Design review of the part shown in the three views and the two pictorial views. Dimensions are in mm from the part's minimum x, y and z. A direction names the side the tool comes from. Give positions to 0.01 mm unless a question says otherwise; leave off trailing zeros. Order: outer loops, then holes, each group sorted by start corner. A loop starts at its lowest first (then second) coordinate and runs counter-clockwise, first axis right, second up. Notation, with made-up numbers: (-24.75, -12.75) - (-9.75, -12.75) arc R7 ccw to (-9.75, -6.75) - close; hole circle Ø5 at (80.25, 79.5). An arc over 180 degrees is marked (long way). Put each result on its own line as item: value.
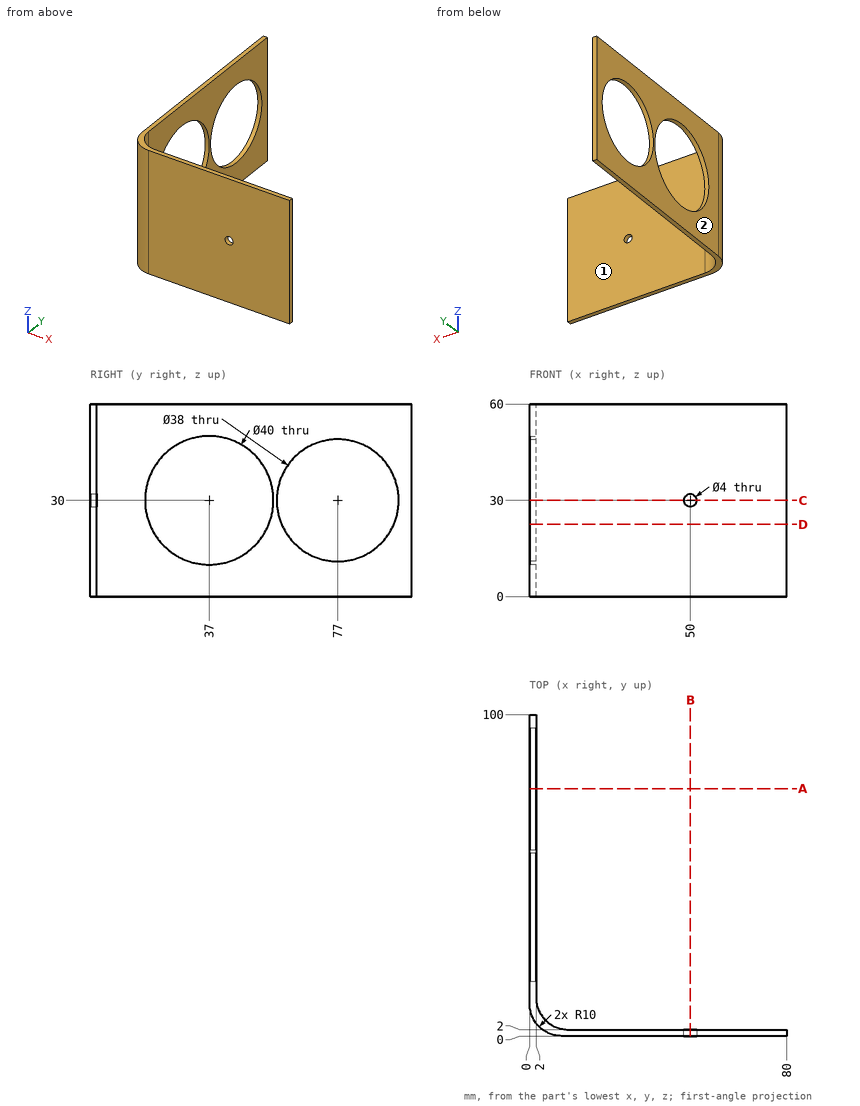
(1) Clearance check with flat-ended pins moving along their axes: pin 1 Ø1.5 at (x, z) = (29, 23) entering from -Y; pin 2 Ø18 at (y, z) = (49.5, 29.5) entering from +X; pin 3 Ø2 at (x, z) = (33, 8.5) entering from +Y. State where each tip first meets the part, or that it passes through.
The answers:
pin 1: y = 0
pin 2: x = 2
pin 3: y = 2
(2) Wall thickness on L1, parallel to Y at x = 1, z = 30; L2, parallel to Y at x = 1.25, z = 30; L3, parallel to Y at x = 14.5, z = 25.5: over which ranges is each line inside the solid? List them lowest first.
The answers:
L1: 5.64 to 17, 57 to 58, 96 to 100
L2: 5.16 to 17, 57 to 58, 96 to 100
L3: 0 to 2
(3) Take a section at A-A, the plane y = 77. Write out the cut boundary in (x, z).
The answers:
outline: (0, 0) - (2, 0) - (2, 11) - (0, 11) - close; (0, 49) - (2, 49) - (2, 60) - (0, 60) - close
(4) Take a section at C-C, the plane z = 30. Write out the cut boundary in (x, y).
The answers:
outline: (0, 10) arc R10 ccw to (10, 0) - (48, 0) - (48, 2) - (12, 2) arc R10 cw to (2, 12) - (2, 17) - (0, 17) - close; (0, 57) - (2, 57) - (2, 58) - (0, 58) - close; (0, 96) - (2, 96) - (2, 100) - (0, 100) - close; (52, 0) - (80, 0) - (80, 2) - (52, 2) - close
(5) Take a section at D-D, the plane z = 22.5. Write out the cut boundary in (x, y), then the cut area to 3 significant figures.
The answers:
outline: (0, 10) arc R10 ccw to (10, 0) - (80, 0) - (80, 2) - (12, 2) arc R10 cw to (2, 12) - (2, 18.46) - (0, 18.46) - close; (0, 55.54) - (2, 55.54) - (2, 59.54) - (0, 59.54) - close; (0, 94.46) - (2, 94.46) - (2, 100) - (0, 100) - close
area: 212 mm^2
(6) For the marked faces 1 and 2, list the 3-axis set-ups (+Z, -Z, +X, -X, +Y, -Y) from which the entire face can be reached by the end or side of a thin tool; tool diameter is ignored.
The answers:
face 1: +Z, -Z, +X, +Y
face 2: +Z, -Z, -X, +Y, -Y
(7) Take a section at B-B, the plane x = 50. Write out the cut boundary in (y, z), then the cut area to 3 significant figures.
The answers:
outline: (0, 0) - (2, 0) - (2, 28) - (0, 28) - close; (0, 32) - (2, 32) - (2, 60) - (0, 60) - close
area: 112 mm^2
